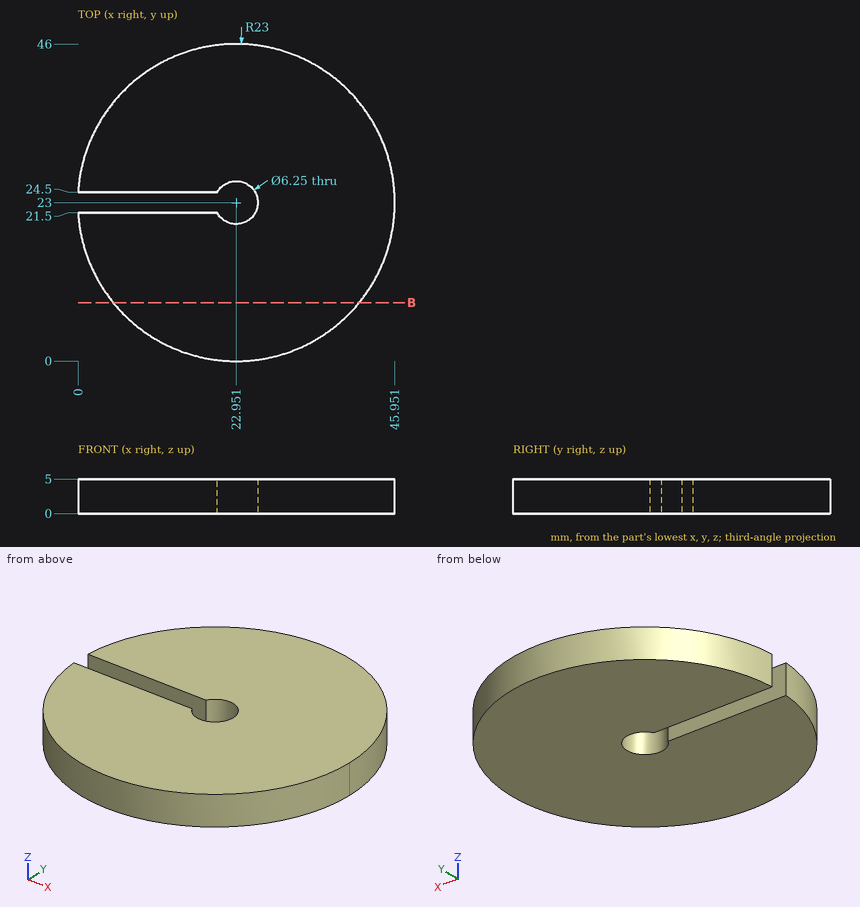
Input: dimensioned drawing with shaded views. Units: mm. Origin: part minimum x, y, z. Round coordinates to 2 decimals unless told otherwise and drop trailing zeros. Loops run counter-clockwise (first coordinate to the right, second up) from the corner with the lowest first, then second, coordinate; pieces in that order, holes last. Notation, with made-up numbers: (87, -16.5) -> (123, -16.5) arc R12 cw to (123, -0.5) -> close; hole circle Ø7 at (19.25, 53.25). An arc over 180 degrees is marked (long way). Answer as a JSON object with one key per item and string values. Group by question number.
Q1. Section query B-B (y = 8.5). Output: boundary loops of the cut face in (x, z).
Q2. Contact query for flat-ended pins moving along their axis: P1, Ø5, axis at x = 19.5, y = 22, coming from the -Z side; P2, Ø2.5, axis at x = 12.5, z = 2.5, coming from the +Y side. Output: stop coordinate, or through.
Q3. Ray query, line 1 (Y direction, x = 23, z = 1.85); line 2 (Y direction, x = 9, z = 3.9); line 3 (X direction, y = 23, z = 3.6). Return the intervals inside material, ascending. Write a range as from..to.
Completed:
{
 "1": {"outline": "(5.1, 0) -> (40.8, 0) -> (40.8, 5) -> (5.1, 5) -> close"},
 "2": {"P1": "z = 0", "P2": "y = 44.08"},
 "3": {"line 1": "0..19.88, 26.12..46", "line 2": "4.71..21.5, 24.5..41.29", "line 3": "26.08..45.95"}
}
